Could you check a few things on this model? Use its own coordinates, in mm. A direction names the side the tool comes from. Give positions to 0.01 mm unless a question says otherwise; leave off trailing zeros. Order: outer loops, then holes, each group sorted by start corner. A loop starts at its lowest first (then second) coordinate and runs counter-clockwise, first axis right, second up.
from build123d import *

# Parameters (mm, degrees)
BOSS_EXTRUDE1_DEPTH = 2
CHAMFER1_SIZE       = 2
SKETCH2_R           = 1.6
CUT_EXTRUDE1_DEPTH  = 103.019605959
CHAMFER2_SIZE       = 2


with BuildPart() as part:
    # Sketch1 → Boss-Extrude1 (new body)
    with BuildSketch(Plane(origin=(0, 0, 0), x_dir=(1, 0, 0), z_dir=(0, 1, 0))):
        Polygon((0, 0), (0, 4), (40, 4), (70, 0), (90, 0), (82, -48), (0, -48), align=None)
    extrude(amount=BOSS_EXTRUDE1_DEPTH)

    # Chamfer1
    chamfer1_edges = [part.edges().sort_by_distance(p)[0] for p in [
        (41, 0, 48),
    ]]
    chamfer(chamfer1_edges, length=CHAMFER1_SIZE - 0.0001)  # a hair under: the kernel refuses the full size

    # Sketch2 → Cut-Extrude1 (cut, through all)
    with BuildSketch(Plane(origin=(0, 2, 0), x_dir=(1, 0, 0), z_dir=(0, 1, 0))):
        with Locations(Location((4, -7, 0), (0, 0, 270))):
            Circle(SKETCH2_R)
        with Locations(Location((4, -29, 0), (0, 0, 270))):
            Circle(SKETCH2_R)
        with Locations(Location((74, -7, 0), (0, 0, 270))):
            Circle(SKETCH2_R)
        with Locations(Location((74, -29, 0), (0, 0, 270))):
            Circle(SKETCH2_R)
    extrude(amount=-CUT_EXTRUDE1_DEPTH, mode=Mode.SUBTRACT)

    # Chamfer2
    chamfer2_edges = [part.edges().sort_by_distance(p)[0] for p in [
        (4, 2, 27.4),
        (74, 2, 5.4),
        (74, 2, 27.4),
        (4, 2, 5.4),
    ]]
    chamfer(chamfer2_edges, length=CHAMFER2_SIZE - 0.0001)  # a hair under: the kernel refuses the full size


solid = part.part
Item 1: For faces 4 (the flat face through (80, 1, 0)), 5 (the flat face through (46, 2, 22)), which set-ups out of +Z, -Z, +X, -X, +Y, -Y let a thin tool reach every point of the face, with its end or its side?
Findings:
face 4: -Z, +X, +Y, -Y
face 5: +Z, -Z, +X, -X, +Y
Item 2: Please list where these lines run through material, in increasing order: line 1 along X through (y, z) = (0.7, 6.5); line 2 along X through (y, z) = (0.05, 7); line 3 along Z through (x, y) = (4, 0.05).
Findings:
line 1: x = 0 to 1.76, 6.24 to 71.76, 76.24 to 88.92
line 2: x = 0 to 2.35, 5.65 to 72.35, 75.65 to 88.83
line 3: z = -4 to 5.35, 8.65 to 27.35, 30.65 to 46.05
Item 3: Imagine slicing it at A-A on x = 4. Give the number of separate pieces and of enclosed holes in the cut face, then the cut area to 3 significant figures.
Findings:
separate pieces: 3
enclosed holes: 0
area: 81.2 mm2
Item 4: Imagine slicing it at C-C on y = 1.25. List the corners of the cut face in (x, z) for me.
Findings:
outline: (0, -4) - (40, -4) - (70, 0) - (90, 0) - (82.12, 47.25) - (0, 47.25) - close; hole circle Ø5.7 at (4, 7); hole circle Ø5.7 at (4, 29); hole circle Ø5.7 at (74, 7); hole circle Ø5.7 at (74, 29)
Item 5: For pin 1 (1.9 mm diameter, centred on x = 4, z = 29, fed in from -Y); pin 2 (1 mm diameter, centred on y = 1.5, z = 25, fed in from +X), each with a flat end and sliding along its axis, tell me the tip position at first contact or that it passes through.
Findings:
pin 1: passes through
pin 2: stops at x = 85.92
Item 6: We'd pull the mould along Z, two halves only. Please class faces 1 (the flat face through (55, 1, -2)), 2 (the flat face through (86, 1, 24)), 3 (the flat face through (46, 0, 21)): +Z half, -Z half, draft (parallel to the pull), parting line (faces both ways), or undercut.
Findings:
face 1: -Z half
face 2: +Z half
face 3: draft
